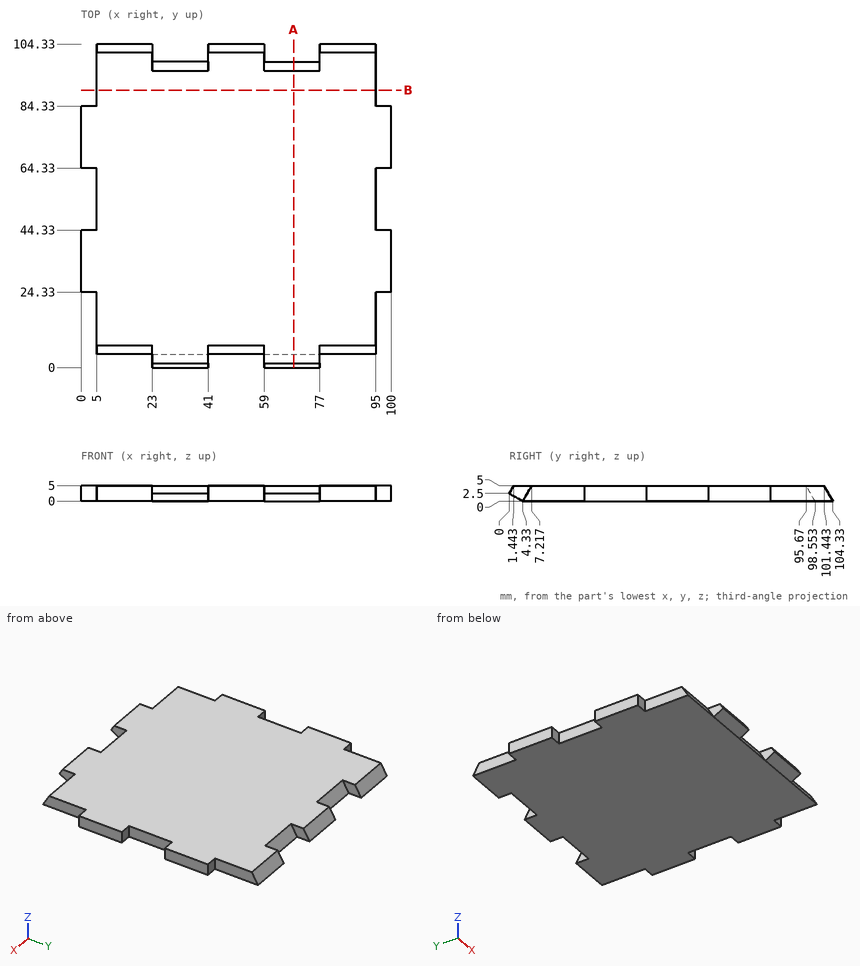
For this review, use the dimensioned drawing (mm, ordinates from the lowest corner) and the shaded views. Coordinates: 2 decimals unless noted, no trailing zeros. Order: outer loops, then holes, each group sorted by start corner. A loop starts at its lowest first (then second) coordinate and runs counter-clockwise, first axis right, second up. Notation, with made-up numbers: (-14.5, -38) - (-8.5, -38) arc R29 ccw to (-8.5, -14) - close; hole circle Ø6 at (-21, 7.25). An arc over 180 degrees is marked (long way). Answer as a JSON object with one key per item and string values. Group by question number.
1. Clearance check with flat-ended pins moving along their axes: P1, Ø1.5, axis at y = 2.5, z = 3.5, coming from the +X side; P2, Ø2, axis at y = 40.5, z = 1, coming from the -X side; P3, Ø2.5, axis at y = 54.5, z = 2, coming from the -X side; P4, Ø2, axis at x = 52, z = 0.5, coming from the +Y side. State where each tip first meets the part, or that it passes through.
2. We need section B-B on y = 89.5. State the section outline as (x, z) points, then the cut area to 3 significant figures.
3. For probe 1 along X at (y, z) = (63.5, 0.8); probe 2 along Y at (x, z) = (88, 4.7) (1 decimal); probe 3 along Y at (x, z) = (35.5, 0.2) (1 decimal), list the stretches that pass through material, from the lowest coordinate up.
4. We need section A-A on x = 68.5. State the section outline as (y, z) points.
Final values:
{
 "1": {"P1": "x = 77", "P2": "x = 0", "P3": "x = 5", "P4": "y = 104.33"},
 "2": {"outline": "(5, 0) - (95, 0) - (95, 5) - (5, 5) - close", "area": "450 mm²"},
 "3": {"probe 1": "5 to 95", "probe 2": "7 to 101.6", "probe 3": "4 to 98.4"},
 "4": {"outline": "(0, 2.5) - (4.33, 0) - (98.55, 0) - (95.67, 5) - (1.44, 5) - close"}
}
